```python
from build123d import *

# Parameters (mm, degrees)
BOSS_EXTRUDE1_DEPTH = 2
BOSS_EXTRUDE2_DEPTH = 3
FILLET1_R           = 3


with BuildPart() as part:
    # Sketch1 → Boss-Extrude1 (new body)
    with BuildSketch(Plane.ZY.offset(329.974562358)):
        with BuildLine():
            Line((137.105001839, 14.690261729), (137.105001839, -0.019509128))
            Line((137.105001839, -0.019509128), (133.705001839, -0.019509128))
            Line((133.705001839, -0.019509128), (129.505001839, -0.019509128))
            Line((129.505001839, -0.019509128), (129.505001839, -17.019509128))
            Line((129.505001839, -17.019509128), (-21.848970599, -17.019509128))
            Line((-21.848970599, -17.019509128), (-21.848970599, -0.019509128))
            Line((-21.848970599, -0.019509128), (-26.048970599, -0.019509128))
            Line((-26.048970599, -0.019509128), (-29.448970599, -0.019509128))
            Line((-29.448970599, -0.019509128), (-29.448970599, 47.708117707))
            ThreePointArc((-29.448970599, 47.708117707), (-28.460366767, 49.843262649), (-26.192653512, 50.470684397))
            Line((-26.192653512, 50.470684397), (74.05116687, 33.912543624))
            Line((74.05116687, 33.912543624), (79.277875997, 26.617509644))
            Line((79.277875997, 26.617509644), (134.761318926, 17.452828418))
            ThreePointArc((134.761318926, 17.452828418), (136.440146781, 16.501657897), (137.105001839, 14.690261729))
        make_face()
    extrude(amount=-BOSS_EXTRUDE1_DEPTH)

    # Sketch1<4> → Boss-Extrude2 (add)
    with BuildSketch(Plane.ZY.offset(329.974562358)):
        with BuildLine():
            Line((140.305001839, -17.219509128), (140.305001839, 17.2353763))
            ThreePointArc((140.305001839, 17.2353763), (139.592657134, 19.176157909), (137.793913004, 20.195269182))
            Line((137.793913004, 20.195269182), (82.333171975, 29.356200538))
            ThreePointArc((82.333171975, 29.356200538), (81.237686153, 29.768607171), (80.383410411, 30.568845492))
            Line((80.383410411, 30.568845492), (76.604168861, 35.843616835))
            ThreePointArc((76.604168861, 35.843616835), (75.749893119, 36.643855156), (74.654407298, 37.056261789))
            Line((74.654407298, 37.056261789), (-29.160059434, 54.204197172))
            ThreePointArc((-29.160059434, 54.204197172), (-31.589752208, 53.531959584), (-32.648970599, 51.24430429))
            Line((-32.648970599, 51.24430429), (-32.648970599, -17.219509128))
            ThreePointArc((-32.648970599, -17.219509128), (-31.770290943, -19.340829471), (-29.648970599, -20.219509128))
            Line((-29.648970599, -20.219509128), (137.305001839, -20.219509128))
            ThreePointArc((137.305001839, -20.219509128), (139.426322182, -19.340829471), (140.305001839, -17.219509128))
        make_face()
    extrude(amount=BOSS_EXTRUDE2_DEPTH)

    # Fillet1
    fillet1_edges = [part.edges().sort_by_distance(p)[0] for p in [
        (-332.974562358, 17.012397581, -32.648970599),
        (-332.974562358, 53.531959584, -31.589752208),
        (-332.974562358, 45.63022948, 22.747173932),
        (-332.974562358, 36.643855156, 75.749893119),
        (-332.974562358, 33.206231163, 78.493789636),
        (-332.974562358, 29.768607171, 81.237686153),
        (-332.974562358, 24.77573486, 110.063542489),
        (-332.974562358, 19.176157909, 139.592657134),
        (-332.974562358, 0.007933586, 140.305001839),
        (-332.974562358, -19.340829471, 139.426322182),
        (-332.974562358, -20.219509128, 53.82801562),
        (-332.974562358, -19.340829471, -31.770290943),
    ]]
    fillet(fillet1_edges, radius=FILLET1_R - 0.0001)  # a hair under: the kernel refuses the full size


with BuildPart() as body_2:
    # Mirror1: mirrored copy
    add(part.part.mirror(Plane.ZY.offset(327.974562358)))


solid = body_2.part
```
Design review of the part built by this model. Coordinates are the model's own, in mm. A direction names the side the tool comes from. Give positions to 0.01 mm unless a question says otherwise; leave off trailing zeros. Write each loop counter-clockwise with the first axis right and the second up, starting at its lowest first coordinate (ties: lowest second). Pieces come first, ordered by that corner, then holes. Notation, with made-up numbers: (-20.75, 25) - (28.25, 25) arc R13 cw to (28.25, 35) - close; hole circle Ø10 at (57, -22). An arc over 180 degrees is marked (long way). Return JSON: item names as keys, results as strings. Group by question number.
(1) Machinability: for faces 1 (the flat face through (-326.96, 22.1, 106.63)), 2 (the cylindrical face through (-323.83, 23.95, 109.53)), which of the approach directions +Z, -Z, +X, -X, +Y, -Y give a long, thin tool a straight path to every point of the face, cutting with its end or side? Answer none if there is none.
(2) To check wall thickness, follow probe 1 along Z at (x, y) = (-326.7, -10) (3 decimals); probe 2 along Z at (x, y) = (-323.5, -3); probe 3 along Y at (x, z) = (-327.05, 97). State the ranges of each line that lie inside material, in increasing order.
(3) Insertion check: pin 1 (1 mm diameter, centred on x = -327, z = 41.5, fed in from -Y); pin 2 (1 mm diameter, centred on x = -327.5, y = 23.5, fed in from -Z); pin 3 (0.6 mm diameter, centred on x = -327, z = -24.5, fed in from -Y). Each pin has a flat end and moves straight along its axis. Give the tip position at first contact, or say it passes through.
(4) We need section B-B, the plane x = -326.95. Give the boundary of the cut face in (y, z) (1 decimal).
Reported:
{
 "1": {"face 1": "+Z, -X, +Y", "face 2": "+Z, +X, +Y"},
 "2": {"probe 1": "z = -21.849 to 129.505", "probe 2": "z = -31.35 to 139", "probe 3": "y = -17.02 to 23.69"},
 "3": {"pin 1": "stops at y = -17.02", "pin 2": "stops at z = -29.45", "pin 3": "stops at y = -0.02"},
 "4": {"outline": "(-17, -21.8) - (0, -21.8) - (0, -29.4) - (47.7, -29.4) arc R2.8 ccw to (50.5, -26.2) - (33.9, 74.1) - (26.6, 79.3) - (17.5, 134.8) arc R2.8 ccw to (14.7, 137.1) - (0, 137.1) - (0, 129.5) - (-17, 129.5) - close"}
}
